Geometry check sheet. Reference: the model listing, model coordinates, mm. A direction names the side the tool comes from. Round coordinates to 2 decimals unless told otherwise and drop trailing zeros. Write each loop counter-clockwise with the first axis right and the second up, starting at its lowest first coordinate (ties: lowest second). Pieces come first, ordered by that corner, then holes. Notation, with made-up numbers: M 84.25,-30.75 L 114.25,-30.75 A22 cw 114.25,-9.75 Z; hole C 59.25,20 d6. An arc over 180 degrees is marked long. Put each result on its own line as item: value. Start each with the question number.
(1) Tool access check on faces 5 (the flat face through (2, -2, 5)), 6 (the flat face through (2, 21, 0.174)). Record the directions out of +Z, -Z, +X, -X, +Y, -Y that give a thin tool (end or side, any length) a straight path to the whole face; none if there is none.
(2) Section check C-C on y = -25. Record the cut outline in (x, z), then the cut area to 3 significant figures.
(3) Material ranges on probe 1 along Z at (x, y) = (2.1, 32); probe 2 along Y at (x, z) = (0.6, 36); probe 3 along Z at (x, y) = (1.35, 15), recorded low to high.
(4) Gauge pin test, flat end, axial feed: pin 1 (1.2 mm diameter, centred on x = 3, z = 4.5, fed in from +Y). Record the tip position at first contact, or that the pin passes through.
(5) Section check A-A on x = 0.65. Record the cut outline in (y, z).
(6) Section check B-B on z = 6. Record the cut outline in (x, y), then the cut area to 3 significant figures.
(7) Section check D-D on z = 20. Record the cut outline in (x, y), then the cut area to 3 significant figures.
(8) Mould release check, pull along Y, two halves, no side actions. Record for faces 1 (the flat face through (2, 2, 5)), 2 (the flat face through (1.97, 20.28, 28.68)), 3 (the flat face through (2, 0, 10.174)), 4 (the flat face through (2, -21, 0.174)): pulls with the +Y half, pulls with the -Y half, needs draft (parallel to the pull), parting line crosses it, or undercut.
from build123d import *

# Parameters (mm, degrees)
PAD_DEPTH = 4


with BuildPart() as part:
    # Sketch → Pad (new body)
    with BuildSketch(Plane.YZ):
        Polygon((0, 58), (-40, 0.173901), (-2, 0.173901), (-2, 10.173901), (2, 10.173901), (2, 0.173901), (40, 0.173901), align=None)
    extrude(amount=PAD_DEPTH)


solid = part.part
Answers follow:
1. face 5: -Z, +X, -X
1. face 6: -Z, +X, -X, +Y, -Y
2. outline: M 0,0.17 L 4,0.17 L 4,21.86 L 0,21.86 Z
2. area: 86.7 mm^2
3. probe 1: z = 0.17 to 11.74
3. probe 2: y = -15.22 to 15.22
3. probe 3: z = 0.17 to 36.32
4. pin 1: stops at y = 37.42
5. outline: M -40,0.17 L -2,0.17 L -2,10.17 L 2,10.17 L 2,0.17 L 40,0.17 L 0,58 Z
6. outline: M 0,-35.97 L 4,-35.97 L 4,-2 L 0,-2 Z; M 0,2 L 4,2 L 4,35.97 L 0,35.97 Z
6. area: 272 mm^2
7. outline: M 0,-26.29 L 4,-26.29 L 4,26.29 L 0,26.29 Z
7. area: 210 mm^2
8. face 1: undercut
8. face 2: pulls with the +Y half
8. face 3: undercut
8. face 4: needs draft
